Geometry: see drawing. Coordinates: mm, zero at the bounding-box minimum. A direction names the side the tool comes from. Round coordinates to 2 decimals unless told otherwise and drop trailing zeros. Order: outer loops, then holes, each group sorted by start corner. A loop starts at its lowest first (then second) coordinate and runs counter-clockwise, first axis right, second up. Notation, with made-up numbers: (41.5, -9) -> (82.5, -9) arc R8 cw to (82.5, 6) -> close; hole circle Ø5 at (32.5, 68). An arc over 180 degrees is marked (long way). Answer as CSV lines item,"result". Start each with the question number.
(1) Set-up query: the marked faces 1, 2 and 3. Return all of +Z, -Z, +X, -X, +Y, -Y with unobstructed straight access to the full face (end or side cutting, diameter ignored); none if empty.
(2) Line query: line 1 along Z through (x, y) = (27, 11.95); line 2 along Y through (x, z) = (30, 2.5); line 3 along Z through (x, y) = (29.5, 6). Output: solid intervals per line, ascending. Write a range as from..to.
(3) Section query D-D (z = 5). Output: boundary loops of the cut face in (x, y).
(4) Pull-direction query (Z, two-part tool) for the marked faces 4, 5 and 6; classes: +Z half, -Z half, draft (parallel to the pull), parting line (faces both ways), or undercut.
(5) Section query A-A (x = 27). Count the separate pieces of the cut face and the enclosed holes in it, plus the area to 3 significant figures.
(6) Contact query for flat-ended pins moving along their axis: P1, Ø4, axis at y = 8, z = 18, coming from the -X side; P2, Ø4.5, axis at x = 27, z = 5, coming from the +Y side; P3, Ø7, axis at x = 28, z = 26.5, coming from the -Y side; P4, Ø3, axis at x = 5, z = 27, coming from the +Y side. Output: stop coordinate, or through.
(7) Section query C-C (x = 5). Output: boundary loops of the cut face in (y, z).
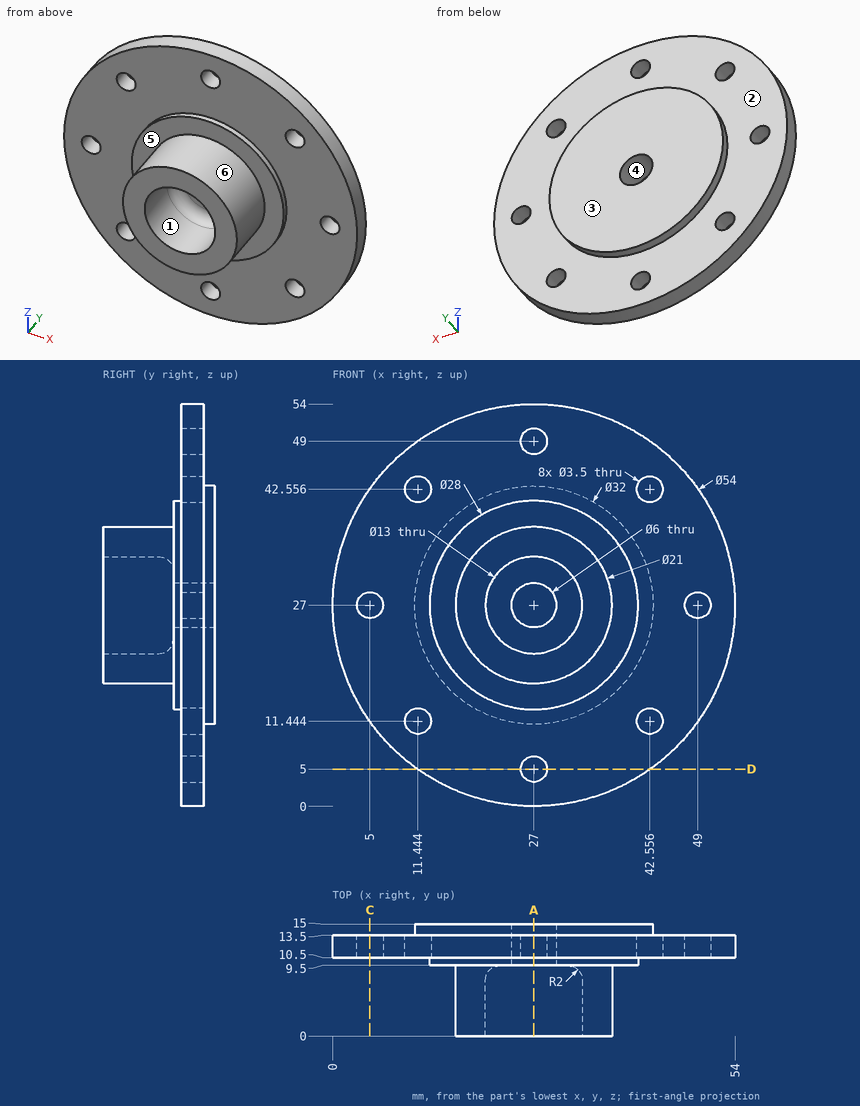
Answer block:
1,face 1,"-Y"
1,face 2,"+Y"
1,face 3,"+Z, -Z, +X, -X, +Y"
2,line 1,"0..3.25, 6.75..24, 30..47.25, 50.75..54"
2,line 2,"10.5..13.5"
2,line 3,"16.8..21, 33..37.2"
3,outline,"(11.35, 10.5) -> (25.25, 10.5) -> (25.25, 13.5) -> (11.35, 13.5) -> close; (28.75, 10.5) -> (42.65, 10.5) -> (42.65, 13.5) -> (28.75, 13.5) -> close"
4,face 4,"undercut"
4,face 5,"draft"
4,face 6,"parting line"
5,separate pieces,"4"
5,enclosed holes,"0"
5,area,"262 mm2"
6,P1,"x = 15.29"
6,P2,"y = 13.5"
6,P3,"y = 9.5"
6,P4,"through"
7,outline,"(10.5, 11.35) -> (13.5, 11.35) -> (13.5, 25.25) -> (10.5, 25.25) -> close; (10.5, 28.75) -> (13.5, 28.75) -> (13.5, 42.65) -> (10.5, 42.65) -> close"
